```python
from build123d import *

# Parameters (mm, degrees)
F0_W     = 120
F0_H     = 120
F1_DEPTH = 2
F2_R     = 2.5
F3_DEPTH = 2.001
F4_R     = 5
F5_DEPTH = 2.001


with BuildPart() as f1:
    # F0 (on Front) → F1 (new body)
    with BuildSketch(Plane.XZ):
        Rectangle(F0_W, F0_H)
    extrude(amount=F1_DEPTH)

    # F2 (on face) → F3 (cut, through all)
    with BuildSketch(Plane.XZ.offset(2)):
        with Locations((-55, 55)):
            Circle(F2_R)
        with Locations((55, -55)):
            Circle(F2_R)
    extrude(amount=-F3_DEPTH, mode=Mode.SUBTRACT)

    # F4 (on face) → F5 (cut, through all)
    with BuildSketch(Plane.XZ.offset(2)):
        Circle(F4_R)
    extrude(amount=-F5_DEPTH, mode=Mode.SUBTRACT)


solid = f1.part
```
Design review of the part built by this model. Coordinates are the model's own, in mm. Give positions to 0.01 mm unless a question says otherwise; leave off trailing zeros. Loops run counter-clockwise (first coordinate to the right, second up) from the corner with the lowest first, then second, coordinate; pieces in that order, holes last. Notation, with made-up numbers: M 4,-19 L 39,-19 A31 cw 39,18 Z; hole C 17.25,23.25 d3. An arc over 180 degrees is marked long. Return JSON: item names as keys, results as strings. Group by question number.
Item 1: Mouldability with a two-part tool opening along X and no side actions: class faces 1 (the flat face through (-1, -2, -12)), 2 (the cylindrical face through (-1.08, -1.01, -4.88)) as released by +X, released by -X, zero draft, split by the parting line, or undercut.
Item 2: We need section A-A (z = -55). Give the boundary of the cut face in (x, y), and give its area (3 significant figures).
Item 3: For probe 1 along Z at (x, y) = (0, -0.6); probe 2 along Z at (x, y) = (-55, -0.85), list the stretches that pass through material, from the lowest coordinate up.
Item 4: We need section B-B (x = 55). Give the boundary of the cut face in (y, z).
Output:
{
 "1": {"face 1": "zero draft", "face 2": "undercut"},
 "2": {"outline": "M -60,-2 L 52.5,-2 L 52.5,0 L -60,0 Z; M 57.5,-2 L 60,-2 L 60,0 L 57.5,0 Z", "area": "230 mm^2"},
 "3": {"probe 1": "z = -60 to -5, 5 to 60", "probe 2": "z = -60 to 52.5, 57.5 to 60"},
 "4": {"outline": "M -2,-60 L 0,-60 L 0,-57.5 L -2,-57.5 Z; M -2,-52.5 L 0,-52.5 L 0,60 L -2,60 Z"}
}
